The figure shows three views and two pictorial views of one solid part (mm, origin at its lowest corner). Answer the questions. Coordinates: 2 decimals unless noted, no trailing zeros. Loops run counter-clockwise (first coordinate to the right, second up) from the corner with the lowest first, then second, coordinate; pieces in that order, holes last. Notation, with made-up numbers: M 60,-39 L 109,-39 A33 cw 109,-11 Z; hole C -29,83 d6. An arc over 180 degrees is marked long. Answer in a Markdown table with one row per item. Add a question column.
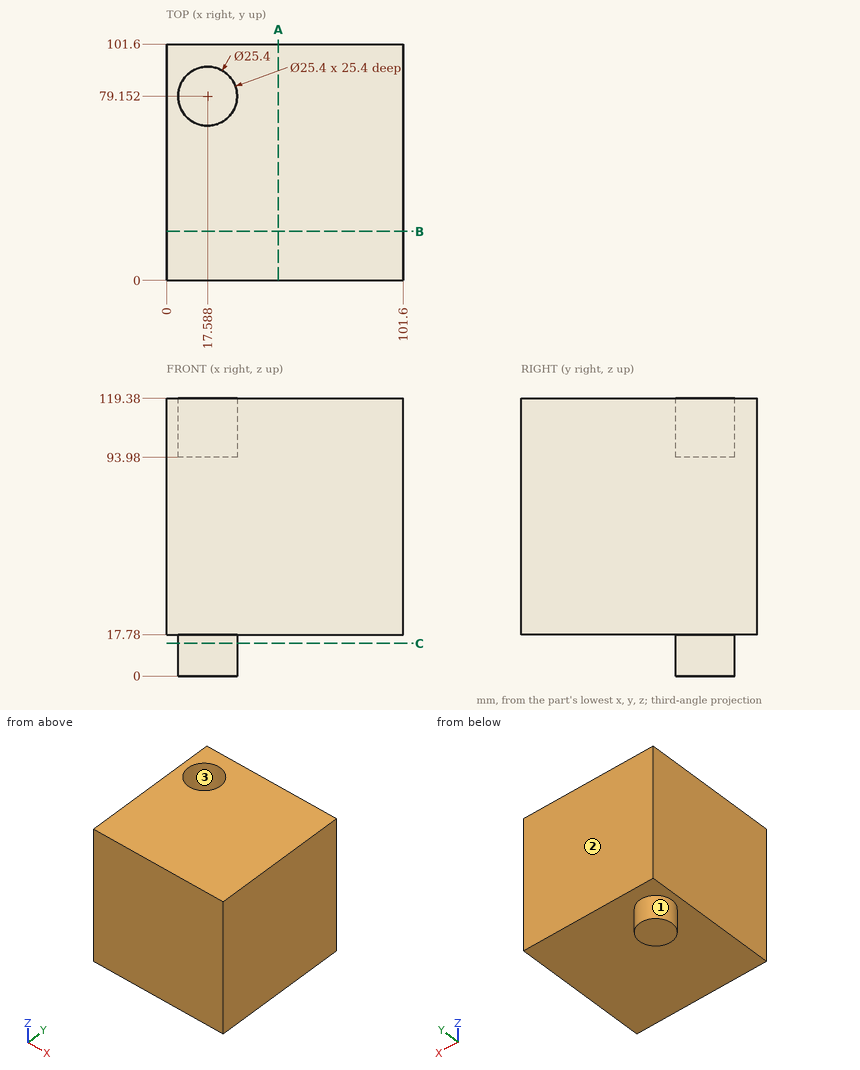
(1) A cutting plane is placed at A-A (x = 48). Give the vertices of the cut face in (y, z), plus the area to 3 significant figures.
(2) Each of these flat-tipped pins is pushed along its axis until it touches: pin 1 (2 mm diameter, centred on y = 16.5, z = 87, fed in from -X); pin 2 (12 mm diameter, centred on x = 56.5, y = 85.5, fed in from -Z). Where does it stop, or does it pass through?
(3) Straight lines are drawn through the part: line 1 (Z direction, x = 46, y = 42.5); line 2 (X direction, y = 76, z = 101) (1 decimal); line 3 (Z direction, x = 27, y = 78.5). For each, find the intervals that lie inside material, in ascending order.
(4) The mould has two halves that part along X. Classify the marked faces 1, 2 and 3: released by +X, released by -X, zero draft, split by the parting line, or undercut.
(5) A cutting plane is placed at C-C (z = 14). Give the vertices of the cut face in (x, y).
Solved:
| question | item | result |
|---|---|---|
| 1 | outline | M 0,17.78 L 101.6,17.78 L 101.6,119.38 L 0,119.38 Z |
| 1 | area | 10,300 mm² |
| 2 | pin 1 | stops at x = 0 |
| 2 | pin 2 | stops at z = 17.78 |
| 3 | line 1 | z = 17.78 to 119.38 |
| 3 | line 2 | x = 0 to 5.3, 29.9 to 101.6 |
| 3 | line 3 | z = 0 to 93.98 |
| 4 | face 1 | split by the parting line |
| 4 | face 2 | zero draft |
| 4 | face 3 | undercut |
| 5 | outline | C 17.59,79.15 d25.4 |
